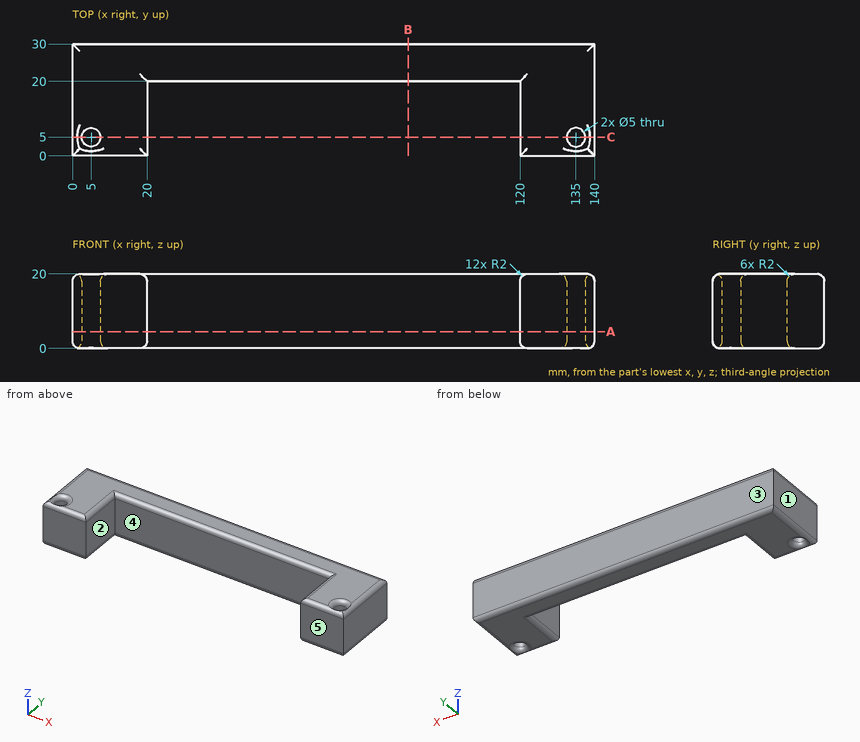
Study the drawing (mm; zero at the part's minimum x, y, z) and answer. A direction names the side the tool comes from. Give positions to 0.01 mm unless a question says otherwise; leave off trailing zeros. Loops run counter-clockwise (first coordinate to the right, second up) from the corner with the lowest first, then second, coordinate; pieces in that order, holes last. Notation, with made-up numbers: M 33.25,-32.5 L 84.25,-32.5 A13 cw 84.25,-15.5 Z; hole C -3.75,-10.5 d9. An arc over 180 degrees is marked long. One line per item, written item: value.
1. Section A-A on z = 4.5 is taken. Determine the outline of the cut face in (x, y).
Found:
outline: M 0,0 L 20,0 L 20,20 L 120,20 L 120,0 L 140,0 L 140,30 L 0,30 Z; hole C 5,5 d5; hole C 135,5 d5
2. Find the intervals of material crossed by probe 1 along Y at (x, z) = (5, 13); probe 2 along X at (y, z) = (4, 11.25); probe 3 along X at (y, z) = (9.5, 10), in increasing order.
Found:
probe 1: 0 to 2.5, 7.5 to 30
probe 2: 0 to 2.71, 7.29 to 20, 120 to 132.71, 137.29 to 140
probe 3: 0 to 20, 120 to 140
3. Each of these flat-tipped pins is pushed along its axis until it touches: P1, Ø6, axis at x = 135, y = 5, coming from the +Z side; P2, Ø4, axis at x = 53, z = 6.5, coming from the -Y side. Where does it stop, or does it pass through?
Found:
P1: z = 19.32
P2: y = 20
4. Section B-B on x = 90 is taken. Determine the outline of the cut face in (y, z).
Found:
outline: M 20,2 A2 ccw 22,0 L 28,0 A2 ccw 30,2 L 30,18 A2 ccw 28,20 L 22,20 A2 ccw 20,18 Z
5. For a pull along X with two mould halves and no side action, classify the marked faces 1, 2 and 3 as pulls with the +X half, pulls with the -X half, needs draft (parallel to the pull), parting line crosses it, or undercut.
Found:
face 1: pulls with the -X half
face 2: undercut
face 3: needs draft
6. Section C-C on y = 5 is taken. State how many separate pieces and enclosed holes the cut face has, plus the area to 3 significant figures.
Found:
separate pieces: 4
enclosed holes: 0
area: 587 mm^2
7. For the marked faces 4 and 5, determine the directions among +Z, -Z, +X, -X, +Y, -Y from which every point of the face is accessible in a straight line to the end or side of a thin tool.
Found:
face 4: +Z, -Z, -Y
face 5: +Z, -Z, +X, -X, -Y
